Source: three-view drawing plus pictorial views. Frame: mm from the lowest corner of the part. A direction names the side the tool comes from. Coordinates: 2 decimals unless noted, no trailing zeros. Write each loop counter-clockwise with the first axis right and the second up, starting at its lowest first coordinate (ties: lowest second). Pieces come first, ordered by that corner, then holes. Notation, with made-up numbers: M -29,70.5 L 22,70.5 A32 cw 22,97.5 Z; hole C 88,41.25 d1. An arc over 180 degrees is marked long. Use CSV: the item, a comma, the result in double quotes.
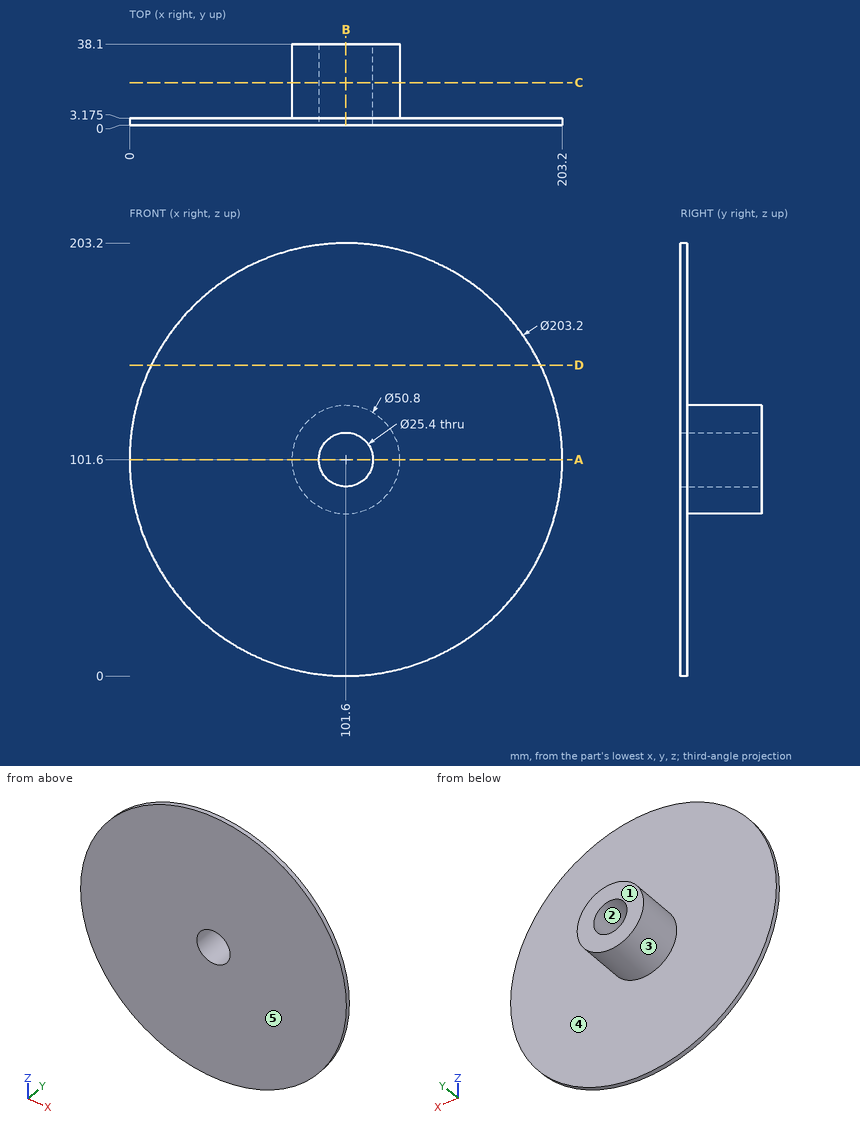
1. Section C-C (y = 20). Return loops of the section in (x, z), then the cut area to 3 significant figures.
Resolved:
outline,"C 101.6,101.6 d50.8; hole C 101.6,101.6 d25.4"
area,"1,520 mm^2"
2. Contact query for flat-ended pins moving along their axis: pin 1 Ø3 at (y, z) = (5.5, 136) entering from -X; pin 2 Ø10 at (y, z) = (32, 125) entering from +X; pin 3 Ø6 at (x, y) = (99, 11.5) entering from -Z; pin 4 Ø10 at (y, z) = (26, 90) entering from -X. Output: stop coordinate, or through.
Resolved:
pin 1,"passes through"
pin 2,"stops at x = 119.11"
pin 3,"stops at z = 76.2"
pin 4,"stops at x = 77.07"
3. Access query for the marked faces 4 and 5. Directions: +Z, -Z, +X, -X, +Y, -Y. A direction counts if a zero-diameter tool reaches every point of the face in a straight line with its end or side. Return the directions, or none.
Resolved:
face 4,"+Y"
face 5,"+Z, -Z, +X, -X, -Y"
4. Material intervals for line 1 (Z direction, x = 101.6, y = 20); line 2 (X direction, y = 25, z = 101); line 3 (Y direction, x = 142, z = 136) (3 decimals), sorted ascending. Write a range as [from, to].
Resolved:
line 1,"z = [76.2, 88.9], [114.3, 127]"
line 2,"x = [76.21, 88.91], [114.29, 126.99]"
line 3,"y = [0, 3.175]"
5. Section A-A (z = 101.6). Return loops of the section in (x, y) (3 decimals).
Resolved:
outline,"M 0,0 L 88.9,0 L 88.9,38.1 L 76.2,38.1 L 76.2,3.175 L 0,3.175 Z; M 114.3,0 L 203.2,0 L 203.2,3.175 L 127,3.175 L 127,38.1 L 114.3,38.1 Z"
6. Section D-D (z = 146). Return loops of the section in (x, y) (3 decimals).
Resolved:
outline,"M 10.215,0 L 192.985,0 L 192.985,3.175 L 10.215,3.175 Z"
7. Mould query, pull axis X, two halves, no side actions, for the marked faces 1, 2 and 3. Classes: pulls with the +X half, pulls with the -X half, needs draft (parallel to the pull), parting line crosses it, or undercut.
Resolved:
face 1,"needs draft"
face 2,"undercut"
face 3,"parting line crosses it"
8. Section B-B (x = 101.6). Return loops of the section in (y, z) (3 decimals).
Resolved:
outline,"M 0,0 L 3.175,0 L 3.175,76.2 L 38.1,76.2 L 38.1,88.9 L 0,88.9 Z; M 0,114.3 L 38.1,114.3 L 38.1,127 L 3.175,127 L 3.175,203.2 L 0,203.2 Z"
